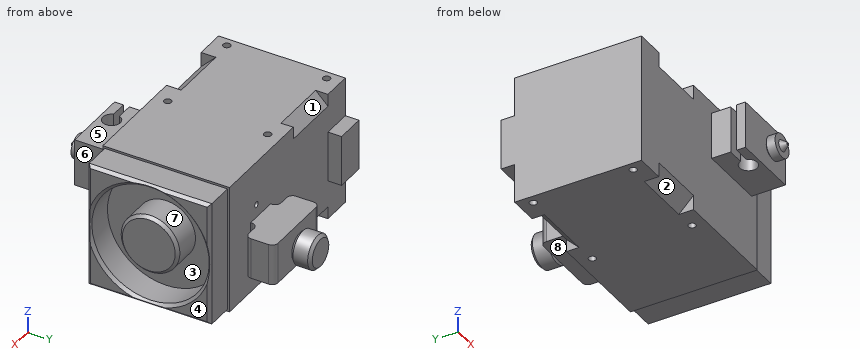
```python
from build123d import *

# Parameters (mm, degrees)
MAIN_BLOCK_SKETCH_W            = 76.75
MAIN_BLOCK_SKETCH_H            = 43.2
MAIN_BLOCK_DEPTH               = 44
HEATER_BLOCK_DEPTH             = 8
JST_CONNECTOR_SKETCH_W         = 17.28
JST_CONNECTOR_SKETCH_H         = 4.64
JST_CONNECTOR_BLOCK_DEPTH      = 10
IDLER_BLOCK_DEPTH              = 14
MOTOR_INSET_CUTOUT_SKETCH_W    = 46
MOTOR_INSET_CUTOUT_SKETCH_H    = 46
MOTOR_INSET_DEPTH              = 20
FAN_SKETCH_R                   = 20
FAN_SKETCH_R_2                 = 10
MAIN_FAN_ROTOR_CUT_DEPTH       = 10
FAN_EDGE_CUT_SKETCH_W          = 50
FAN_EDGE_CUT_SKETCH_H          = 49.09090909
FAN_EDGE_CUT_SKETCH_W_2        = 42.57287206
FAN_EDGE_CUT_SKETCH_H_2        = 41.79881984
FAN_HOUSING_CUT_DEPTH          = 10
MOUNTING_HOLES_NEAR_SIDE_D     = 2.5
MOUNTING_HOLES_NEAR_SIDE_DEPTH = 3
MOUNTING_HOLES_NEAR_SIDE_TIP   = 0.751075774
MOUNTING_HOLES_FAR_SIDE_D      = 2.5
MOUNTING_HOLES_FAR_SIDE_DEPTH  = 3
MOUNTING_HOLES_FAR_SIDE_TIP    = 0.751075774
FILAMENT_HOLE_D                = 2
FILAMENT_HOLE_DEPTH            = 10
FILAMENT_HOLE_TIP              = 0.600860619
COSMETIC_CHAMFERS_SIZE         = 1
TENSION_ARM_FILLETS_R          = 2
NOZZLE_FILLET_R                = 0.2


with BuildPart() as part:
    # Main Block Sketch → Main Block (new body)
    with BuildSketch(Plane.XY):
        with Locations((35.375, 17)):
            Rectangle(MAIN_BLOCK_SKETCH_W, MAIN_BLOCK_SKETCH_H)
    extrude(amount=-MAIN_BLOCK_DEPTH)


with BuildPart() as body_2:
    # Nozzle +Heatbreak Sketch → Nozzle+heatbreak (revolve)
    with BuildSketch(Plane.XY.offset(-15.1), mode=Mode.PRIVATE) as nozzle_heatbreak_sk:
        Polygon((48.25, -11.7), (48.25, -23.5), (48.45, -23.5), (48.45, -24.2), (48.75, -24.2), (50.150415076, -22.2), (52.25, -22.2), (52.25, -19.2), (51.25, -19.2), (51.25, -11.7), (50.3, -11.7), (50.3, -4.6), (50.3, -3.6), (48.25, -3.6), (48.25, -4.6), align=None)
    revolve(nozzle_heatbreak_sk.sketch.rotate(Axis((48.25, 38.6, -15.1), (0, -1, 0)), 180), axis=Axis((48.25, 38.6, -15.1), (0, -1, 0)))

    # Heater Block Sketch → Heater Block (add, symmetric)
    with BuildSketch(Plane.XY.offset(-15.1)):
        with BuildLine():
            Line((38.921572875, -13.6), (33.25, -13.6))
            Line((33.25, -13.6), (33.25, -7.1))
            Line((33.25, -7.1), (56.25, -7.1))
            Line((56.25, -7.1), (56.25, -18.6))
            Line((56.25, -18.6), (33.25, -18.6))
            Line((33.25, -18.6), (33.25, -15.6))
            Line((33.25, -15.6), (38.921572875, -15.6))
            ThreePointArc((38.921572875, -15.6), (44.75, -14.6), (38.921572875, -13.6))
        make_face()
    extrude(amount=HEATER_BLOCK_DEPTH, both=True)


with BuildPart() as body_3:
    # JST Connector Sketch → JST Connector Block (new body)
    with BuildSketch(Plane(origin=(-3, 0, 0), x_dir=(0, 0, -1), z_dir=(1, 0, 0))):
        with Locations((22, 40.92)):
            Rectangle(JST_CONNECTOR_SKETCH_W, JST_CONNECTOR_SKETCH_H)
    extrude(amount=JST_CONNECTOR_BLOCK_DEPTH)


with BuildPart() as body_4:
    # Idler Block Sketch → Idler Block (new body)
    with BuildSketch(Plane.XY.offset(-19.5)):
        Polygon((40.05, 38.6), (40.05, 41), (32.85, 41), (32.85, 51), (58.75, 51), (58.75, 41), (51.55, 41), (51.55, 38.6), align=None)
    extrude(amount=-IDLER_BLOCK_DEPTH)


with BuildPart() as body_5:
    # Tension knob sketch → Tension Knob (revolve)
    with BuildSketch(Plane.XY.offset(-26.5), mode=Mode.PRIVATE) as tension_knob_sk:
        Polygon((46.8, 52), (46.8, 49), (45.8, 49), (45.8, 52), (45.8, 59), (51.55, 59), (51.55, 52), align=None)
    revolve(tension_knob_sk.sketch.rotate(Axis((45.8, 59, -26.5), (0, -1, 0)), 90), axis=Axis((45.8, 59, -26.5), (0, -1, 0)))

    # Combination of Parts: union body 4, body 3, body 2, part
    add(body_4.part)
    add(body_3.part)
    add(body_2.part)
    add(part.part)

    # Motor Inset Cutout Sketch → Motor Inset (cut)
    with BuildSketch(Plane(origin=(7, 0, 0), x_dir=(0, 0, -1), z_dir=(1, 0, 0))):
        with Locations((22, 17.4)):
            Rectangle(MOTOR_INSET_CUTOUT_SKETCH_W, MOTOR_INSET_CUTOUT_SKETCH_H)
        Polygon((5, 39.4), (39, 39.4), (44, 34.4), (44, 0.4), (39, -4.6), (5, -4.6), (0, 0.4), (0, 34.4), align=None, mode=Mode.SUBTRACT)
    extrude(amount=MOTOR_INSET_DEPTH, mode=Mode.SUBTRACT)

    # Fan Sketch → Main Fan Rotor Cut (cut)
    with BuildSketch(Plane(origin=(73.75, 0, 0), x_dir=(0, 0, -1), z_dir=(1, 0, 0))):
        with Locations((22, 17)):
            Circle(FAN_SKETCH_R)
        with Locations((22, 17)):
            Circle(FAN_SKETCH_R_2, mode=Mode.SUBTRACT)
    extrude(amount=-MAIN_FAN_ROTOR_CUT_DEPTH, mode=Mode.SUBTRACT)

    # Fan Edge Cut Sketch → Fan Housing Cut (cut)
    with BuildSketch(Plane(origin=(73.75, 0, 0), x_dir=(0, 0, -1), z_dir=(1, 0, 0))):
        with Locations((22, 17)):
            Rectangle(FAN_EDGE_CUT_SKETCH_W, FAN_EDGE_CUT_SKETCH_H)
        with Locations((22, 17)):
            Rectangle(FAN_EDGE_CUT_SKETCH_W_2, FAN_EDGE_CUT_SKETCH_H_2, mode=Mode.SUBTRACT)
    extrude(amount=-FAN_HOUSING_CUT_DEPTH, mode=Mode.SUBTRACT)

    # Mounting Holes Near Side
    with Locations(Plane.XY):
        with Locations((0, 34), (0, 0), (34, 0), (34, 34)):
            Hole(MOUNTING_HOLES_NEAR_SIDE_D / 2, depth=MOUNTING_HOLES_NEAR_SIDE_DEPTH)
            with Locations((0, 0, -(MOUNTING_HOLES_NEAR_SIDE_DEPTH + MOUNTING_HOLES_NEAR_SIDE_TIP / 2))):  # 118° drill point
                Cone(0, MOUNTING_HOLES_NEAR_SIDE_D / 2, MOUNTING_HOLES_NEAR_SIDE_TIP, mode=Mode.SUBTRACT)

    # Mounting Holes Far Side
    with Locations(Plane(origin=(0, 0, -44), x_dir=(1, 0, 0), z_dir=(0, 0, -1))):
        with Locations((0, 0), (34, 0), (34, -34), (0, -34)):
            Hole(MOUNTING_HOLES_FAR_SIDE_D / 2, depth=MOUNTING_HOLES_FAR_SIDE_DEPTH)
            with Locations((0, 0, -(MOUNTING_HOLES_FAR_SIDE_DEPTH + MOUNTING_HOLES_FAR_SIDE_TIP / 2))):  # 118° drill point
                Cone(0, MOUNTING_HOLES_FAR_SIDE_D / 2, MOUNTING_HOLES_FAR_SIDE_TIP, mode=Mode.SUBTRACT)

    # Filament Hole
    with Locations(Plane(origin=(0, 38.6, 0), x_dir=(1, 0, 0), z_dir=(0, 1, 0))):
        with Locations((48.228258832, 15.029737369)):
            Hole(FILAMENT_HOLE_D / 2, depth=FILAMENT_HOLE_DEPTH)
            with Locations((0, 0, -(FILAMENT_HOLE_DEPTH + FILAMENT_HOLE_TIP / 2))):  # 118° drill point
                Cone(0, FILAMENT_HOLE_D / 2, FILAMENT_HOLE_TIP, mode=Mode.SUBTRACT)

    # Cosmetic Chamfers
    # the kernel refuses this chamfer: 1 mm, written as the material it adds along each edge
    with BuildSketch(Plane(origin=(48.25, -4.6, -15.1), x_dir=(-1, 0, 0), z_dir=(0, 0, -1))) as cosmetic_chamfers_piece_1:
        Polygon((2.05 + COSMETIC_CHAMFERS_SIZE, 0), (2.05, -COSMETIC_CHAMFERS_SIZE), (2.05, 0), align=None)
    revolve(axis=Axis((48.25, -4.6, -15.1), (0, 1, 0)))
    # the kernel refuses this chamfer: 1 mm, written as the material it takes off along each edge
    with BuildSketch(Plane(origin=(73.75, 17, -22), x_dir=(0, 0, -1), z_dir=(0, -1, 0))) as cosmetic_chamfers_2_piece_1:
        Polygon((20 + COSMETIC_CHAMFERS_SIZE, 0), (20, -COSMETIC_CHAMFERS_SIZE), (20, 0), align=None)
    revolve(axis=Axis((73.75, 17, -22), (1, 0, 0)), mode=Mode.SUBTRACT)
    with BuildSketch(Plane(origin=(73.75, 17, -22), x_dir=(0, 0, -1), z_dir=(0, -1, 0))) as cosmetic_chamfers_2_piece_2:
        Polygon((10, -COSMETIC_CHAMFERS_SIZE), (10 - COSMETIC_CHAMFERS_SIZE, 0), (10, 0), align=None)
    revolve(axis=Axis((73.75, 17, -22), (1, 0, 0)), mode=Mode.SUBTRACT)
    with BuildSketch(Plane(origin=(73.75, 37.89940992, 1.858119018), x_dir=(-0.9996219169112968, 0.027495876610589196, 0), z_dir=(0, 0, -1)), Plane(origin=(73.75, -3.89940992, -45.858119018), x_dir=(-0.9996219169112968, -0.027495876610586605, 0), z_dir=(0, 0, 1))) as cosmetic_chamfers_2_piece_3:
        Polygon((COSMETIC_CHAMFERS_SIZE * 0.999621916911, -COSMETIC_CHAMFERS_SIZE * 0.0274958766106), (-COSMETIC_CHAMFERS_SIZE * 0.0274958766106, -COSMETIC_CHAMFERS_SIZE * 0.999621916911), (0, 0), align=None)
    extrude(amount=47.716238035, mode=Mode.SUBTRACT)
    with BuildSketch(Plane(origin=(73.75, -6.471092908, -0.71356397), x_dir=(-0.9996219169112968, 0, 0.027495876610586497), z_dir=(0, 1, 0)), Plane(origin=(73.75, 40.471092908, -43.28643603), x_dir=(-0.9996219169112968, 0, -0.027495876610589196), z_dir=(0, -1, 0))) as cosmetic_chamfers_2_piece_4:
        Polygon((COSMETIC_CHAMFERS_SIZE * 0.999621916911, -COSMETIC_CHAMFERS_SIZE * 0.0274958766106), (-COSMETIC_CHAMFERS_SIZE * 0.0274958766106, -COSMETIC_CHAMFERS_SIZE * 0.999621916911), (0, 0), align=None)
    extrude(amount=46.942185816, mode=Mode.SUBTRACT)
    with BuildSketch(Plane(origin=(45.8, 52, -26.5), x_dir=(0, 0, 1), z_dir=(1, 0, 0))) as cosmetic_chamfers_2_piece_5:
        Polygon((5.75 - COSMETIC_CHAMFERS_SIZE, 0), (5.75, -COSMETIC_CHAMFERS_SIZE), (5.75, 0), align=None)
    revolve(axis=Axis((45.8, 52, -26.5), (0, -1, 0)), mode=Mode.SUBTRACT)
    with BuildSketch(Plane(origin=(45.8, 59, -26.5), x_dir=(0, 0, 1), z_dir=(1, 0, 0))) as cosmetic_chamfers_2_piece_6:
        Polygon((5.75, COSMETIC_CHAMFERS_SIZE), (5.75 - COSMETIC_CHAMFERS_SIZE, 0), (5.75, 0), align=None)
    revolve(axis=Axis((45.8, 59, -26.5), (0, -1, 0)), mode=Mode.SUBTRACT)

    # Tension Arm Fillets
    tension_arm_fillets_edges = [body_5.edges().sort_by_distance(p)[0] for p in [
        (40.05, 41, -26.5),
        (32.85, 41, -26.5),
        (32.85, 51, -26.5),
        (58.75, 51, -26.5),
        (58.75, 41, -26.5),
        (51.55, 41, -26.5),
    ]]
    fillet(tension_arm_fillets_edges, radius=TENSION_ARM_FILLETS_R)

    # Nozzle Fillet
    nozzle_fillet_edges = [body_5.edges().sort_by_distance(p)[0] for p in [
        (48.75, -24.2, -15.1),
    ]]
    fillet(nozzle_fillet_edges, radius=NOZZLE_FILLET_R)


solid = body_5.part
```
Source: CAD feature listing. Evaluate the final solid. Frame: model axes, mm. Face numbers are marked on the shaded views. A direction names the side the tool comes from. Give positions to 0.01 mm unless a question says otherwise; leave off trailing zeros. Loops run counter-clockwise (first coordinate to the right, second up) from the corner with the lowest first, then second, coordinate; pieces in that order, holes last. Notation, with made-up numbers: (30.25, 83) -> (68.25, 83) arc R19 ccw to (68.25, 105) -> close; hole circle Ø7 at (-39.75, 11.5). An arc over 180 degrees is marked (long way). Use a Markdown table: item, result. Add a question column.
(1) Ray query, line 1 (X direction, y = 34, z = -42); line 2 (Y direction, x = 0, z = -42); line 3 (Y direction, x = 41.75, z = -15.25). Return the intervals inside material, ascending.
(2) Pull-direction query (Y, two-part tool) for the marked faces 1, 2, 3 and 4; classes: +Y half, -Y half, draft (parallel to the pull), parting line (faces both ways), or undercut.
(3) Section query A-A (y = -14.6). Output: boundary loops of the cut face in (x, z).
(4) First-contact query: pin 1 Ø1.5 at (x, y) = (24.5, 41) entering from -Z; pin 2 Ø13 at (x, z) = (31, -15) entering from +Y; pin 3 Ø2 at (x, y) = (53.5, -15) entering from -Z; pin 4 Ø2.5 at (x, y) = (66, 23.5) entering from +Z. Flat tips, straight axial feed; report the tip coordinate or a pass-through.
(5) Access query for the marked faces 5, 6, 7 and 8. Directions: +Z, -Z, +X, -X, +Y, -Y. A direction counts if a zero-diameter tool reaches every point of the face in a straight line with its end or side. Return the directions, or none.
Checked values:
| question | item | result |
|---|---|---|
| 1 | line 1 | -3 to -1.25, 1.25 to 32.75, 35.25 to 73.75 |
| 1 | line 2 | -4.6 to -1.25, 1.25 to 32.75, 35.25 to 38.6 |
| 1 | line 3 | -18.6 to -17.6, -11.6 to -7.1, -4.6 to 38.6 |
| 2 | face 1 | +Y half |
| 2 | face 2 | -Y half |
| 2 | face 3 | undercut |
| 2 | face 4 | draft |
| 3 | outline | (44.75, -23.1) -> (56.25, -23.1) -> (56.25, -7.1) -> (44.75, -7.1) -> close |
| 4 | pin 1 | through |
| 4 | pin 2 | y = 51 |
| 4 | pin 3 | z = -23.1 |
| 4 | pin 4 | z = -0.71 |
| 5 | face 5 | +Z, +X, -X, -Y |
| 5 | face 6 | +Z, -Z, +X, -Y |
| 5 | face 7 | +X |
| 5 | face 8 | -Z, +X, -X, +Y |
